```python
from build123d import *

# Parameters (mm, degrees)
F0_W     = 44.45
F0_H     = 2082.8
F1_DEPTH = 44.45


with BuildPart() as f1:
    # F0 (on Front) → F1 (new body, symmetric)
    with BuildSketch(Plane.XZ):
        with Locations((1031.875, 266.447886)):
            Rectangle(F0_W, F0_H)
        with Locations((22.225, 266.447886)):
            Rectangle(F0_W, F0_H)
        Polygon((0, 1307.847886), (44.45, 1307.847886), (1009.65, 1307.847886), (1054.1, 1307.847886), (1054.1, 1352.297886), (527.05, 1352.297886), (0, 1352.297886), align=None)
    extrude(amount=F1_DEPTH, both=True)


solid = f1.part
```
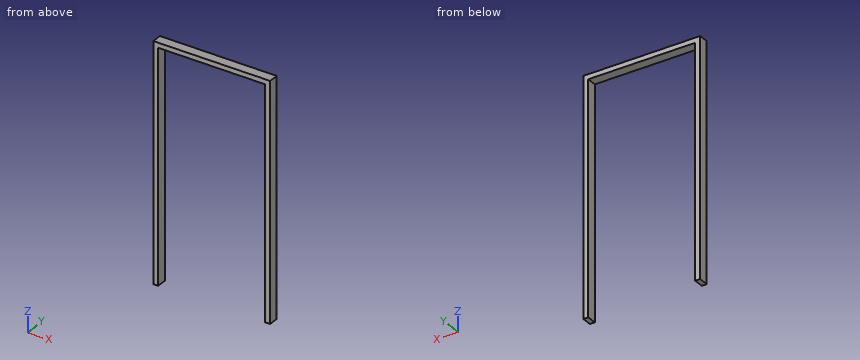
Source: CAD feature listing. Evaluate the final solid. Frame: model axes, mm. Round coordinates to 2 decimals unless told otherwise and drop trailing zeros. Loops run counter-clockwise (first coordinate to the right, second up) from the corner with the lowest first, then second, coordinate; pieces in that order, holes last. Notation, with made-up numbers: M 60,-31 L 80,-31 A22 ccw 80,-19 Z; hole C 25,-5.5 d5. An arc over 180 degrees is marked long. Put each result on its own line as item: value.
(1) Ray query, line 1 (X direction, y = 33.5, z = 111); line 2 (Z direction, x = 730.5, y = 7.5). Return the intervals inside material, ascending. Write a range as [from, to].
Solutions:
line 1: [0, 44.45], [1009.65, 1054.1]
line 2: [1307.85, 1352.3]
(2) Section A-A, the plane z = 374.5. Return loops of the section in (x, y), and give its area (3 significant figures).
Solutions:
outline: M 0,-44.45 L 44.45,-44.45 L 44.45,44.45 L 0,44.45 Z; M 1009.65,-44.45 L 1054.1,-44.45 L 1054.1,44.45 L 1009.65,44.45 Z
area: 7,900 mm²
(3) Section C-C, the plane x = 206.5. Return loops of the section in (y, z).
Solutions:
outline: M -44.45,1307.85 L 44.45,1307.85 L 44.45,1352.3 L -44.45,1352.3 Z
(4) Section B-B, the plane y = -27. Return loops of the section in (x, z).
Solutions:
outline: M 0,-774.95 L 44.45,-774.95 L 44.45,1307.85 L 1009.65,1307.85 L 1009.65,-774.95 L 1054.1,-774.95 L 1054.1,1352.3 L 0,1352.3 Z
